from build123d import *

# Parameters (mm, degrees)
SKETCH1_W           = 36
SKETCH1_H           = 36
SKETCH1_W_2         = 20
SKETCH1_H_2         = 20
BOSS_EXTRUDE4_DEPTH = 35
SKETCH9_W           = 50
SKETCH9_H           = 50
SKETCH9_W_2         = 22
SKETCH9_H_2         = 22
BOSS_EXTRUDE6_DEPTH = 5
SKETCH10_R          = 1.75
CUT_EXTRUDE2_DEPTH  = 10
CUT_EXTRUDE3_DEPTH  = 10
SKETCH4_W           = 40
SKETCH4_H           = 40
BOSS_EXTRUDE7_DEPTH = 10
SKETCH12_R          = 3
CUT_EXTRUDE4_DEPTH  = 4
CHAMFER1_SIZE       = 1
SKETCH13_R          = 1.75
CUT_EXTRUDE5_DEPTH  = 13
CUT_EXTRUDE7_DEPTH  = 2.4


with BuildPart() as part:
    # Sketch1 → Boss-Extrude4 (new body)
    with BuildSketch(Plane(origin=(0, 0, 0), x_dir=(1, 0, 0), z_dir=(0, 1, 0))):
        Rectangle(SKETCH1_W, SKETCH1_H)
        Rectangle(SKETCH1_W_2, SKETCH1_H_2, mode=Mode.SUBTRACT)
    extrude(amount=BOSS_EXTRUDE4_DEPTH)

    # Sketch9 → Boss-Extrude6 (add)
    with BuildSketch(Plane(origin=(0, 30, 0), x_dir=(1, 0, 0), z_dir=(0, 1, 0))):
        Rectangle(SKETCH9_W, SKETCH9_H)
        Rectangle(SKETCH9_W_2, SKETCH9_H_2, mode=Mode.SUBTRACT)
    extrude(amount=BOSS_EXTRUDE6_DEPTH)

    # Sketch10 → Cut-Extrude2 (cut)
    with BuildSketch(Plane(origin=(0, 25, 0), x_dir=(1, 0, 0), z_dir=(0, 1, 0))):
        with Locations((-21.25, 21.25)):
            Circle(SKETCH10_R)
        with Locations((21.25, 21.25)):
            Circle(SKETCH10_R)
        with Locations((21.25, -21.25)):
            Circle(SKETCH10_R)
        with Locations((-21.25, -21.25)):
            Circle(SKETCH10_R)
    extrude(amount=CUT_EXTRUDE2_DEPTH, mode=Mode.SUBTRACT)

    # Sketch11 → Cut-Extrude3 (cut)
    with BuildSketch(Plane(origin=(0, 25, 0), x_dir=(1, 0, 0), z_dir=(0, 1, 0))):
        Polygon((11, 18), (-11, 18), (-18, 25), (18, 25), align=None)
        Polygon((18, 11), (18, -11), (25, -18), (25, 18), align=None)
        Polygon((11, -18), (-11, -18), (-18, -25), (18, -25), align=None)
        Polygon((-18, 11), (-18, -11), (-25, -18), (-25, 18), align=None)
    extrude(amount=CUT_EXTRUDE3_DEPTH, mode=Mode.SUBTRACT)

    # Sketch4 → Boss-Extrude7 (add)
    with BuildSketch(Plane(origin=(0, -5, 0), x_dir=(1, 0, 0), z_dir=(0, 1, 0))):
        Rectangle(SKETCH4_W, SKETCH4_H)
        Polygon((-2.5, -8.548100716), (-2.5, -10), (-10, -10), (-10, -2.5), (-8.422351936, -2.5), (-4.844140472, -8.569430344), align=None, mode=Mode.SUBTRACT)
        Polygon((7.534421013, 0), (3.767210506, 6.525), (-3.767210506, 6.525), (-7.534421013, 0), (-3.767210506, -6.525), (3.767210506, -6.525), align=None, mode=Mode.SUBTRACT)
        Polygon((10, 10), (2.5, 10), (2.5, 8.548100716), (4.844140472, 8.569430344), (8.422351936, 2.5), (10, 2.5), align=None, mode=Mode.SUBTRACT)
        Polygon((10, -10), (2.5, -10), (2.5, -8.502605089), (4.999274138, -8.47986388), (8.379580585, -2.5), (10, -2.5), align=None, mode=Mode.SUBTRACT)
        Polygon((-10, 10), (-10, 2.5), (-8.379580585, 2.5), (-4.999274138, 8.47986388), (-2.5, 8.502605089), (-2.5, 10), align=None, mode=Mode.SUBTRACT)
    extrude(amount=BOSS_EXTRUDE7_DEPTH)

    # Sketch12 → Cut-Extrude4 (cut)
    with BuildSketch(Plane(origin=(0, 35, 0), x_dir=(1, 0, 0), z_dir=(0, 1, 0))):
        with Locations((-14, 14)):
            Circle(SKETCH12_R)
        with Locations((14, 14)):
            Circle(SKETCH12_R)
        with Locations((-14, -14)):
            Circle(SKETCH12_R)
        with Locations((14, -14)):
            Circle(SKETCH12_R)
    extrude(amount=-CUT_EXTRUDE4_DEPTH, mode=Mode.SUBTRACT)

    # Chamfer1
    chamfer1_edges = [part.edges().sort_by_distance(p)[0] for p in [
        (11, 35, -14),
        (-17, 35, 14),
        (11, 35, 14),
        (-17, 35, -14),
    ]]
    chamfer(chamfer1_edges, length=CHAMFER1_SIZE)

    # Sketch13 → Cut-Extrude5 (cut)
    with BuildSketch(Plane(origin=(0, 31, 0), x_dir=(1, 0, 0), z_dir=(0, 1, 0))):
        with Locations((-14, 14)):
            Circle(SKETCH13_R)
        with Locations((14, 14)):
            Circle(SKETCH13_R)
        with Locations((14, -14)):
            Circle(SKETCH13_R)
        with Locations((-14, -14)):
            Circle(SKETCH13_R)
    extrude(amount=-CUT_EXTRUDE5_DEPTH, mode=Mode.SUBTRACT)

    # Sketch15 → Cut-Extrude7 (cut)
    with BuildSketch(Plane(origin=(0, 18, 0), x_dir=(1, 0, 0), z_dir=(0, 1, 0))):
        Polygon((-10.766838493, 14), (-12.383419246, 16.8), (-15.581535205, 22.339299329), (-24.484943605, 19.967960566), (-22.149680093, 11.2), (-15.616580754, 11.2), (-12.383419246, 11.2), align=None)
        Polygon((15.616580754, 11.2), (12.383419246, 11.2), (10.766838493, 14), (12.383419246, 16.8), (15.581535205, 22.339299329), (24.484943605, 19.967960566), (22.149680093, 11.2), align=None)
        Polygon((15.616580754, -11.2), (12.383419246, -11.2), (10.766838493, -14), (12.383419246, -16.8), (15.581535205, -22.339299329), (24.484943605, -19.967960566), (22.149680093, -11.2), align=None)
        Polygon((-15.616580754, -11.2), (-12.383419246, -11.2), (-10.766838493, -14), (-12.383419246, -16.8), (-15.581535205, -22.339299329), (-24.484943605, -19.967960566), (-22.149680093, -11.2), align=None)
    extrude(amount=CUT_EXTRUDE7_DEPTH, mode=Mode.SUBTRACT)


solid = part.part
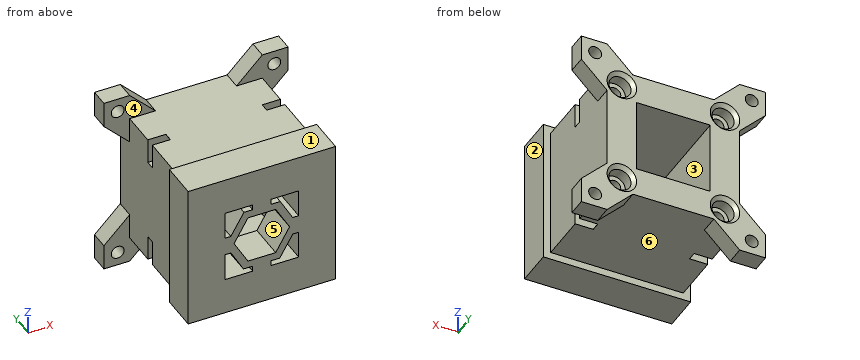
Design review of the part built by this model. Coordinates are the model's own, in mm. Face numbers are marked on the shaded views. A direction names the side the tool comes from. Coordinates: 2 decimals unless noted, no trailing zeros. Order: outer loops, then holes, each group sorted by start corner. A loop starts at its lowest first (then second) coordinate and runs counter-clockwise, first axis right, second up. Notation, with made-up numbers: (36, 45.5) -> (46, 45.5) arc R22 cw to (46, 64.5) -> close; hole circle Ø6 at (87.25, -18.5). An arc over 180 degrees is marked (long way). One line per item, written item: value.
1) Draft analysis for pull direction Z (two halves, no side actions). For the marked faces 4, 5 and 6, state which applies: +Z half, -Z half, draft (parallel to the pull), parting line (faces both ways), or undercut.
Output values:
face 4: draft
face 5: undercut
face 6: -Z half
2) We need section A-A, the plane z = 21.25. Give the boundary of the cut face in (x, y), then the cut area to 3 significant figures.
Output values:
outline: (-25, 30) -> (-23, 30) -> (-23, 35) -> (-25, 35) -> close; (-19.5, 30) -> (-14.25, 30) -> (-14.25, 35) -> (-19.5, 35) -> close; (14.25, 30) -> (19.5, 30) -> (19.5, 35) -> (14.25, 35) -> close; (23, 30) -> (25, 30) -> (25, 35) -> (23, 35) -> close
area: 72.5 mm2
3) To check wall thickness, follow probe 1 along Z at (x, y) = (-14, 27.5); probe 2 along Y at (x, z) = (-19, 14). State the ranges of each line that lie inside material, in increasing order. Write a range as [from, to].
Output values:
probe 1: z = [-18, -15.75], [-12.25, 12.25], [15.75, 18]
probe 2: y = [-5, 5], [30, 35]
4) We need section D-D, the plane y = 10. Give the boundary of the cut face in (x, z), then the cut area to 3 significant figures.
Output values:
outline: (-18, -18) -> (18, -18) -> (18, 18) -> (-18, 18) -> close; hole (-10, -10) -> (10, -10) -> (10, 10) -> (-10, 10) -> close
area: 896 mm2
5) Machinability: for the marked faces 1, 2 and 3, which of the approach directions +Z, -Z, +X, -X, +Y, -Y give a long, thin tool a straight path to every point of the face, cutting with its end or side? Answer none if there is none.
Output values:
face 1: +Z, +X, -X, -Y
face 2: +Z, -Z, +X, -Y
face 3: +Y
6) We need section B-B, the plane x = 21.25. Give the boundary of the cut face in (y, z).
Output values:
outline: (30, -25) -> (35, -25) -> (35, -23) -> (30, -23) -> close; (30, -19.5) -> (35, -19.5) -> (35, -14.25) -> (30, -14.25) -> close; (30, 14.25) -> (35, 14.25) -> (35, 19.5) -> (30, 19.5) -> close; (30, 23) -> (35, 23) -> (35, 25) -> (30, 25) -> close
7) We need section C-C, the plane y = 27. Give the boundary of the cut face in (x, z).
Output values:
outline: (-18, -18) -> (18, -18) -> (18, 18) -> (-18, 18) -> close; hole circle Ø3.5 at (-14, -14); hole circle Ø3.5 at (-14, 14); hole (-10, -10) -> (10, -10) -> (10, 10) -> (-10, 10) -> close; hole circle Ø3.5 at (14, -14); hole circle Ø3.5 at (14, 14)
8) Clearance check with flat-ended pins moving along their axes: P1, Ø5, axis at y = 0.5, z = 2.5, coming from the +X side; P2, Ø3.5, axis at x = 13.5, z = -15.5, coming from the +Y side; P3, Ø1.5, axis at y = 22.5, z = 16, coming from the +X side; P4, Ø8, axis at x = 3.5, z = 4, coming from the -Y side. State where each tip first meets the part, or that it passes through.
Output values:
P1: stops at x = 20
P2: stops at y = 34.33
P3: stops at x = 18
P4: stops at y = -5
